The model under review builds one solid part; all positions refer to its coordinate system, in mm. Face numbers are marked on the shaded views. A direction names the side the tool comes from. Give positions to 0.01 mm unless a question says otherwise; leave off trailing zeros. Loops run counter-clockwise (first coordinate to the right, second up) from the corner with the lowest first, then second, coordinate; pieces in that order, holes last. Notation, with made-up numbers: (81.25, 38) - (130.25, 38) arc R10 ccw to (130.25, 51) - close; hole circle Ø3 at (69, -10.5). An arc over 180 degrees is marked (long way). Answer as a JSON object with one key per item and string values.
from build123d import *

# Parameters (mm, degrees)
SKETCH1_W           = 355.6
SKETCH1_H           = 635
BOSS_EXTRUDE1_DEPTH = 406.4
SHELL1_T            = -6.35
SKETCH2_W           = 165.1
SKETCH2_H           = 152.4
CUT_EXTRUDE1_DEPTH  = 7.35
SKETCH3_R           = 12.7
CUT_EXTRUDE2_DEPTH  = 636


with BuildPart() as part:
    # Sketch1 → Boss-Extrude1 (new body)
    with BuildSketch(Plane(origin=(0, 0, 0), x_dir=(1, 0, 0), z_dir=(0, 1, 0))):
        with Locations((177.8, 317.5)):
            Rectangle(SKETCH1_W, SKETCH1_H)
    extrude(amount=BOSS_EXTRUDE1_DEPTH)

    # Shell1
    shell1_openings = [part.faces().sort_by_distance(p)[0] for p in [
        (177.8, 406.4, -317.5),
        (177.8, 0, -317.5),
        (355.6, 203.2, -317.5),
    ]]
    offset(amount=SHELL1_T, openings=shell1_openings, kind=Kind.INTERSECTION)

    # Sketch2 → Cut-Extrude1 (cut, through all)
    with BuildSketch(Plane(origin=(6.35, 0, 0), x_dir=(0, 0, -1), z_dir=(1, 0, 0))):
        with Locations((463.55, 76.2)):
            Rectangle(SKETCH2_W, SKETCH2_H)
    extrude(amount=-CUT_EXTRUDE1_DEPTH, mode=Mode.SUBTRACT)

    # Sketch3 → Cut-Extrude2 (cut, through all)
    with BuildSketch(Plane.XY):
        with Locations((311.15, 107.95)):
            Circle(SKETCH3_R)
    extrude(amount=-CUT_EXTRUDE2_DEPTH, mode=Mode.SUBTRACT)


solid = part.part
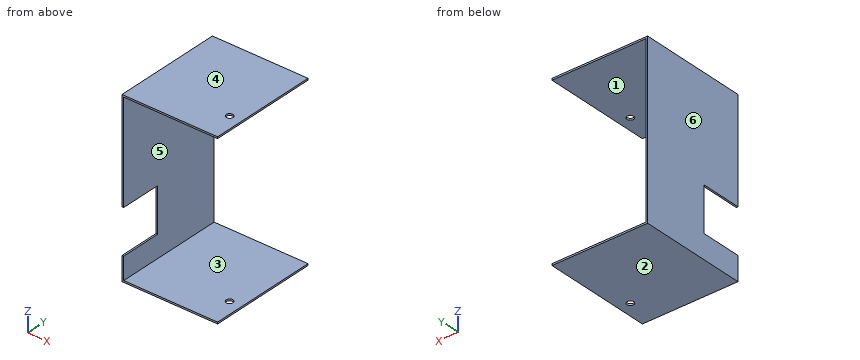
Q1. The part is to be moulded in two halves that separate along Z. For the marked faces 1, 2, 3 and 4, say which applies: +Z half, -Z half, draft (parallel to the pull), parting line (faces both ways), or undercut.
Results:
{"face 1": "undercut", "face 2": "-Z half", "face 3": "undercut", "face 4": "+Z half"}
Q2. For the marked faces 5 and 6, list the 3-axis set-ups (+Z, -Z, +X, -X, +Y, -Y) from which the entire face can be reached by the end or side of a thin tool; tool diameter is ignored.
Results:
{"face 5": "+X, +Y, -Y", "face 6": "+Z, -Z, -X, +Y, -Y"}
Q3. Consider section D-D, the plane y = 171. State the section outline as (x, z) points.
Results:
{"outline": "(0, -635) - (355.6, -635) - (355.6, -628.65) - (6.35, -628.65) - (6.35, -6.35) - (355.6, -6.35) - (355.6, 0) - (0, 0) - close"}
Q4. To check wall thickness, follow probe 1 along Z at (x, y) = (94.5, 300.5); probe 2 along Y at (x, z) = (311, -630). State the ranges of each line that lie inside material, in increasing order. Write a range as [from, to].
Results:
{"probe 1": "z = [-635, -628.65], [-6.35, 0]", "probe 2": "y = [0, 95.25], [120.65, 406.4]"}
Q5. Consider section A-A, the plane x = 186. State the section outline as (y, z) points, plus the area to 3 significant figures.
Results:
{"outline": "(0, -635) - (406.4, -635) - (406.4, -628.65) - (0, -628.65) - close; (0, -6.35) - (406.4, -6.35) - (406.4, 0) - (0, 0) - close", "area": "5,160 mm^2"}
Q6. Consider section C-C, the plane x = 311.15. State the section outline as (y, z) points, plus the area to 3 significant figures.
Results:
{"outline": "(0, -635) - (95.25, -635) - (95.25, -628.65) - (0, -628.65) - close; (0, -6.35) - (95.25, -6.35) - (95.25, 0) - (0, 0) - close; (120.65, -635) - (406.4, -635) - (406.4, -628.65) - (120.65, -628.65) - close; (120.65, -6.35) - (406.4, -6.35) - (406.4, 0) - (120.65, 0) - close", "area": "4,840 mm^2"}
Q7. Consider section B-B, the plane y = 107.95. State the section outline as (x, z) points.
Results:
{"outline": "(0, -635) - (298.45, -635) - (298.45, -628.65) - (6.35, -628.65) - (6.35, -546.1) - (0, -546.1) - close; (0, -381) - (6.35, -381) - (6.35, -6.35) - (298.45, -6.35) - (298.45, 0) - (0, 0) - close; (323.85, -635) - (355.6, -635) - (355.6, -628.65) - (323.85, -628.65) - close; (323.85, -6.35) - (355.6, -6.35) - (355.6, 0) - (323.85, 0) - close"}
Q8. Clearance check with flat-ended pins moving along their axes: pin 1 Ø7 at (x, z) = (3.5, -487.5) entering from -Y; pin 2 Ø3 at (y, z) = (260.5, -184) entering from +X. State where each tip first meets the part, or that it passes through.
Results:
{"pin 1": "stops at y = 152.4", "pin 2": "stops at x = 6.35"}
